```python
from build123d import *

# Parameters (mm, degrees)
F0_W     = 25
F0_H     = 40
F1_DEPTH = 12
F2_R     = 2.5
F3_DEPTH = 123.8
F4_R     = 5
F5_R     = 5
F6_R     = 5
F7_R     = 5
F8_SIZE  = 1


with BuildPart() as f1:
    # F0 (on Top) → F1 (new body)
    with BuildSketch(Plane.XY):
        Rectangle(F0_W, F0_H)
    extrude(amount=F1_DEPTH)

    # F2 (on face) → F3 (cut)
    with BuildSketch(Plane(origin=(0, 0, 0), x_dir=(1, 0, 0), z_dir=(0, 0, -1))):
        with Locations((0, -0.633842)):
            Circle(F2_R)
    extrude(amount=-F3_DEPTH, mode=Mode.SUBTRACT)

    # F4
    f4_edges = [f1.edges().sort_by_distance(p)[0] for p in [
        (-12.5, -20, 6),
    ]]
    fillet(f4_edges, radius=F4_R)

    # F5
    f5_edges = [f1.edges().sort_by_distance(p)[0] for p in [
        (12.5, -20, 6),
    ]]
    fillet(f5_edges, radius=F5_R)

    # F6
    f6_edges = [f1.edges().sort_by_distance(p)[0] for p in [
        (-12.5, 20, 6),
    ]]
    fillet(f6_edges, radius=F6_R)

    # F7
    f7_edges = [f1.edges().sort_by_distance(p)[0] for p in [
        (12.5, 20, 6),
    ]]
    fillet(f7_edges, radius=F7_R)

    # F8
    f8_edges = [f1.edges().sort_by_distance(p)[0] for p in [
        (0, 20, 12),
    ]]
    chamfer(f8_edges, length=F8_SIZE)


solid = f1.part
```
CAD build for the part. Positions are in the model's coordinates, mm. Round coordinates to 2 decimals unless told otherwise and drop trailing zeros. Loops run counter-clockwise (first coordinate to the right, second up) from the corner with the lowest first, then second, coordinate; pieces in that order, holes last. Notation, with made-up numbers: M 49.5,-39 L 81.5,-39 A10 ccw 81.5,-22 Z; hole C 24.25,-13 d11. An arc over 180 degrees is marked long. Use a Markdown table: item, result. Add a question column.
(1) Pull direction Y, two halves, no side cores. Call faces 1 (the face through (12, 0.2, 11.5)), 2 (the face through (1.3, -1.5, 5.9)), 3 (the face through (10.49, 18.05, 11.73)): +Y half, -Y half, draft (parallel to the pull), parting line (faces both ways), or undercut.
(2) Cut at A-A (x = 0). Give the cut face in (y, z).
(3) Cut at B-B (y = 2). Give the cut face in (x, z), and give its area (3 significant figures).
(4) Cut at C-C (z = 1.5). Give the cut face in (x, y), and give its area (3 significant figures).
(5) Drill centre lines: line 1 (Y direction, x = 0, z = 7.5); line 2 (X direction, y = 1, z = 4.25); line 3 (X direction, y = -0.5, z = 5.5). Where is each one in solid material? Low to high.
Geometry says:
| question | item | result |
|---|---|---|
| 1 | face 1 | draft |
| 1 | face 2 | undercut |
| 1 | face 3 | +Y half |
| 2 | outline | M -20,0 L -1.87,0 L -1.87,12 L -19,12 L -20,11 Z; M 3.13,0 L 20,0 L 20,11 L 19,12 L 3.13,12 Z |
| 3 | outline | M -12.5,0 L -2.09,0 L -2.09,12 L -11.5,12 L -12.5,11 Z; M 2.09,0 L 12.5,0 L 12.5,11 L 11.5,12 L 2.09,12 Z |
| 3 | area | 249 mm² |
| 4 | outline | M -12.5,-15 A5 ccw -7.5,-20 L 7.5,-20 A5 ccw 12.5,-15 L 12.5,15 A5 ccw 7.5,20 L -7.5,20 A5 ccw -12.5,15 Z; hole C 0,0.63 d5 |
| 4 | area | 959 mm² |
| 5 | line 1 | y = -20 to -1.87, 3.13 to 20 |
| 5 | line 2 | x = -12.5 to -2.47, 2.47 to 12.5 |
| 5 | line 3 | x = -12.5 to -2.23, 2.23 to 12.5 |
